from build123d import *

# Parameters (mm, degrees)
F0_W     = 127.5
F0_H     = 103.5
F1_DEPTH = 37
F2_R     = 15
F3_W     = 15
F3_H     = 38
F4_DEPTH = 23
F6_DEPTH = 5
F7_R     = 12.5
F8_DEPTH = 95
F9_DEPTH = 2


with BuildPart() as f1:
    # F0 (on Front) → F1 (new body)
    with BuildSketch(Plane.XZ):
        with Locations((63.75, 51.75)):
            Rectangle(F0_W, F0_H)
    extrude(amount=F1_DEPTH)

    # F2
    f2_edges = [f1.edges().sort_by_distance(p)[0] for p in [
        (127.5, -18.5, 103.5),
        (0, -18.5, 103.5),
        (127.5, -18.5, 0),
        (0, -18.5, 0),
    ]]
    fillet(f2_edges, radius=F2_R)

    # F3 (on face) → F4 (join)
    with BuildSketch(Plane.YZ.offset(127.5)):
        with Locations((-18.5, 51.75)):
            Rectangle(F3_W, F3_H)
    extrude(amount=F4_DEPTH)

    # F5 (on face) → F6 (join)
    with BuildSketch(Plane.XZ.offset(37)):
        with BuildLine():
            add(Edge.make_bspline(
                [(97.211815, 51.75), (97.211815, 87.752968), (47.019092, 69.751484), (-3.173631, 51.75), (47.019092, 33.748516), (97.211815, 15.747032), (97.211815, 51.75)],
                knots=[0, 0, 0, 2.094395, 2.094395, 4.18879, 4.18879, 6.283185, 6.283185, 6.283185], degree=2, weights=[1, 0.5, 1, 0.5, 1, 0.5, 1]))
        make_face()
    extrude(amount=F6_DEPTH)

    # F7 (on face) → F8 (join)
    with BuildSketch(Plane.XZ.offset(42)):
        with Locations((47.5, 51.75)):
            Circle(F7_R)
    extrude(amount=-F8_DEPTH)

    # F7 (on face) → F9 (join)
    with BuildSketch(Plane.XZ.offset(42)):
        with Locations((47.5, 51.75)):
            Circle(F7_R)
    extrude(amount=F9_DEPTH)


solid = f1.part
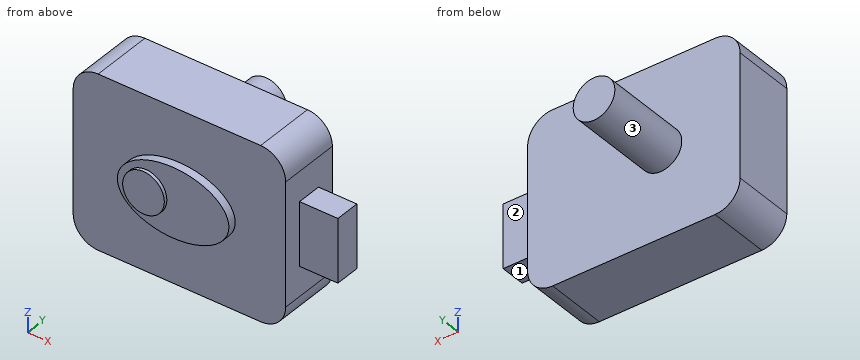
Can you work these out from the model? Positions are in its coordinate system, mm. Face numbers are marked on the shaded views. A direction names the side the tool comes from. Round coordinates to 2 decimals unless told otherwise and drop trailing zeros. Write each loop counter-clockwise with the first axis right and the second up, starting at its lowest first coordinate (ties: lowest second). Pieces come first, ordered by that corner, then holes. Notation, with made-up numbers: M 68,-19 L 108,-19 A19 ccw 108,18 Z; hole C -8.75,34.5 d5. An arc over 180 degrees is marked long. Use a Markdown table: item, result.
Item 1: I want a section at A-A (z = 18). List the corners of the cut face in (x, y) for me, and give its area (3 significant figures).
Found:
| item | result |
|---|---|
| outline | M 0,-37 L 127.5,-37 L 127.5,0 L 0,0 Z |
| area | 4,720 mm2 |
Item 2: For pin 1 Ø4 at (x, z) = (86.5, 81) entering from +Y; pin 2 Ø7.5 at (x, y) = (136.5, -16.5) entering from -Z; pin 3 Ø5 at (x, z) = (102, 47) entering from -Y, each with a flat end and sliding along its axis, tell me the tip position at first contact or that it passes through.
Found:
| item | result |
|---|---|
| pin 1 | stops at y = 0 |
| pin 2 | stops at z = 32.75 |
| pin 3 | stops at y = -37 |
Item 3: I want a section at C-C (x = 110). List the corners of the cut face in (y, z) for me, and give its area (3 significant figures).
Found:
| item | result |
|---|---|
| outline | M -37,0 L 0,0 L 0,103.5 L -37,103.5 Z |
| area | 3,830 mm2 |
Item 4: I want a section at B-B (y = 36). List the corners of the cut face in (x, z) for me.
Found:
| item | result |
|---|---|
| outline | C 47.5,51.75 d25 |
Item 5: Which directions (+Z, -Z, +X, -X, +Y, -Y) give clear straight access to the entire face, cutting with the end or side of a thin tool? Please do the marked faces 1, 2 and 3.
Found:
| item | result |
|---|---|
| face 1 | -Z, +X, +Y, -Y |
| face 2 | +Z, -Z, +X, +Y |
| face 3 | +Y |
Item 6: If I drill on line 1 along Y through (x, z) = (97.5, 91); line 2 along X through (y, z) = (-1, 67); line 3 along Y through (x, z) = (130.5, 38.5), over which ranges is the centre line in solid material (lowest first)? Write a range as [from, to].
Found:
| item | result |
|---|---|
| line 1 | y = [-37, 0] |
| line 2 | x = [0, 127.5] |
| line 3 | y = [-26, -11] |
